Build history of the part. All positions in model axes, mm. Face numbers are marked on the shaded views. Give positions to 0.01 mm unless a question says otherwise; leave off trailing zeros. Write each loop counter-clockwise with the first axis right and the second up, starting at its lowest first coordinate (ties: lowest second). Pieces come first, ordered by that corner, then holes. Notation, with made-up numbers: (8, 5.25) - (34, 5.25) arc R14 ccw to (34, 17.25) - close; hole circle Ø1 at (-37.75, -15.75). An arc over 180 degrees is marked (long way). Use one line per item in the form item = value. Start each with the question number.
Autodesk Inventor part; units mm, degrees
ref_plane "nut_to_pad_XY" through (0, 0, 0) normal (1, 0, 0) x (0, 0, -1)
ref_plane "nut_to_pad_YZ" through (0, 0, 0) normal (0, 0, -1) x (0, 1, 0)
ref_plane "nut_to_pad_ZX" through (0, 0, 0) normal (0, 1, 0) x (1, 0, 0)
sketch "Sketch_1" plane through (0, 0, 0) normal (0, 0, 1) x (1, 0, 0)
  line L0 (4, 0) -> (0, 0)
  line L1 (0, 2.5) -> (0.433, 2.067)
  line L2 (0.433, 2.067) -> (3.567, 2.067)
  line L3 (3.567, 2.067) -> (4, 2.5)
  line L4 (4, 2.5) -> (4, 5)
  line L5 (4, 5) -> (0.6154, 5)
  line L6 (0.6154, 5) -> (0, 3.3333)
  line L7 (0, 3.3333) -> (0, 2.5)
revolve "Revolution1" add sketch "Sketch_1" angle 360 about axis through (4, 0, 0) along (1, 0, 0)
thread "Thread1"
sketch "Sketch_2" plane through (0, 0, 0) normal (1, 0, 0) x (0, 1, 0)
  line L0 (-4.6188, 8) -> (-9.2376, 0)
  line L1 (-9.2376, 0) -> (-4.6188, -8)
  line L2 (-4.6188, -8) -> (4.6188, -8)
  line L3 (4.6188, -8) -> (9.2376, 0)
  line L4 (9.2376, 0) -> (4.6188, 8)
  line L5 (4.6188, 8) -> (-4.6188, 8)
  line L6 (-2.3094, 4) -> (-4.6188, 0)
  line L7 (-4.6188, 0) -> (-2.3094, -4)
  line L8 (-2.3094, -4) -> (2.3094, -4)
  line L9 (2.3094, -4) -> (4.6188, 0)
  line L10 (4.6188, 0) -> (2.3094, 4)
  line L11 (2.3094, 4) -> (-2.3094, 4)
extrude "Extrusion1" cut sketch "Sketch_2" along normal blind 4
ref_plane "nut_to_pad_XY" through (0, 0, 0) normal (1, 0, 0) x (0, 0, -1)
ref_plane "nut_to_pad_YZ" through (0, 0, 0) normal (0, 0, -1) x (0, 1, 0)
ref_plane "nut_to_pad_ZX" through (0, 0, 0) normal (0, 1, 0) x (1, 0, 0)
properties part number "NFJN5nut"
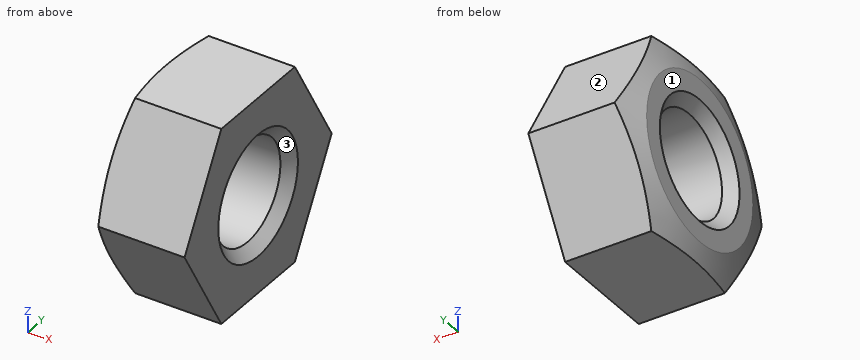
(1) Wall check: line 1 (Z direction, x = 2.9, y = 0); line 2 (Y direction, x = 2.5, z = 1.5); line 3 (Z direction, x = 2.1, y = 0.75). Give the ranges that are in metal, low to high. Write a range as from..to.
(2) Two-plate mould, pull along Y, no slides. Class the marked faces 1, 2 and 3: +Y half, -Y half, draft (parallel to the pull), parting line (faces both ways), or undercut.
(3) Cut at A-A, the plane y = 0. Give the cut face in (x, z), then the cut area to 3 significant figures.
(4) Cut at B-B, the plane x = 1.4. Give the cut face in (y, z), then the cut area to 3 significant figures.
Solution:
q1.line_1 = -4..-2.07, 2.07..4
q1.line_2 = -3.75..-1.42, 1.42..3.75
q1.line_3 = -4..-1.93, 1.93..4
q2.face_1 = draft
q2.face_2 = +Y half
q2.face_3 = undercut
q3.outline = (0, -3.33) - (0.25, -4) - (4, -4) - (4, -2.5) - (3.57, -2.07) - (0.43, -2.07) - (0, -2.5) - close; (0, 2.5) - (0.43, 2.07) - (3.57, 2.07) - (4, 2.5) - (4, 4) - (0.25, 4) - (0, 3.33) - close
q3.area = 14.9 mm2
q4.outline = (-4.62, 0) - (-2.31, -4) - (2.31, -4) - (4.62, 0) - (2.31, 4) - (-2.31, 4) - close; hole circle Ø4.13 at (0, 0)
q4.area = 42.0 mm2
